The model under review builds one solid part; all positions refer to its coordinate system, in mm. A direction names the side the tool comes from. Round coordinates to 2 decimals unless told otherwise and drop trailing zeros. Loops run counter-clockwise (first coordinate to the right, second up) from the corner with the lowest first, then second, coordinate; pieces in that order, holes last. Notation, with made-up numbers: M 42,-17.5 L 47,-17.5 A27 ccw 47,-1.5 Z; hole C 25.5,51.25 d2. An arc over 180 degrees is marked long. Return JSON: item names as keys, results as strings. Group by question number.
Q1. For faces 1 (the face through (-14, 22.5, 0)), 2 (the face through (-11.5, 10, 0)), 3 (the face through (-3.32, 28.7, 0.95)), list the 3-axis set-ups (+Z, -Z, +X, -X, +Y, -Y) from which the entire face can be reached by the end or side of a thin tool; tool diameter is ignored.
Q2. To check wall thickness, follow line 1 along Y through (x, z) = (-0.5, -1.25); line 2 along X through (y, z) = (15, 4); line 3 along Y through (x, z) = (-13.5, -5.5). State the ranges of each line that lie inside material, in increasing order.
Q3. Clearance check with flat-ended pins moving along their axes: pin 1 Ø2 at (x, z) = (-14.5, -3) entering from -Y; pin 2 Ø3.5 at (y, z) = (24.5, -2) entering from -X; pin 3 Ø3.5 at (x, z) = (-12.5, 1) entering from +Y. State where each tip first meets the part, or that it passes through.
Q4. Consider section D-D (y = 18.5). State the section outline as (x, z) points, and give its area (3 significant figures).
Q5. Consider section C-C (z = 0). State the section outline as (x, y) points (3 decimals), and give its area (3 significant figures).
Q6. Consider section B-B (x = -6.35). State the section outline as (y, z) points (3 decimals).
Q7. Consider section A-A (z = 5). State the section outline as (x, y) points.
Autodesk Inventor part; units mm, degrees
ref_plane "YZ Plane" through (0, 0, 0) normal (1, 0, 0) x (0, 1, 0)
ref_plane "XZ Plane" through (0, 0, 0) normal (0, 1, 0) x (-1, 0, 0)
ref_plane "XY Plane" through (0, 0, 0) normal (0, 0, 1) x (1, 0, 0)
sketch "Sketch1" plane through (0, 0, 0) normal (0, 1, 0) x (-1, 0, 0)
  line L0 (11.5, -6) -> (-11.5, -6)
  line L1 (-11.5, -6) -> (-11.5, 6)
  line L2 (-11.5, 6) -> (11.5, 6)
  line L3 (11.5, 6) -> (11.5, -6)
  line L4 (11.5, -6) -> (-11.5, 6) construction
  line L5 (-11.5, -6) -> (11.5, 6) construction
  point P0 (0, 0)
  dimension "d0" = 23
  dimension "d1" = 12
extrude "Extrusion1" add sketch "Sketch1" along normal blind 19.5
sketch "Sketch2" plane through (0, 19.5, 0) normal (0, 1, 0) x (1, 0, 0)
  line L0 (16, -6) -> (-16, -6)
  line L1 (-16, -6) -> (-16, 6)
  line L2 (-16, 6) -> (16, 6)
  line L3 (16, 6) -> (16, -6)
  line L4 (16, -6) -> (-16, 6) construction
  line L5 (-16, -6) -> (16, 6) construction
  point P0 (0, 0)
  dimension "d4" = 32
  dimension "d5" = 12
extrude "Extrusion2" add sketch "Sketch2" along normal blind 3
sketch "Sketch3" plane through (0, 22.5, 0) normal (0, 1, 0) x (1, 0, 0)
  line L0 (11.5, 6) -> (16, 6)
  line L1 (-11.5, -6) -> (11.5, -6)
  line L2 (11.5, -6) -> (11.5, 6)
  line L3 (11.5, 6) -> (-11.5, 6)
  line L4 (-11.5, 6) -> (-11.5, -6)
  line L5 (-11.5, -6) -> (11.5, 6) construction
  line L6 (11.5, -6) -> (-11.5, 6) construction
  point P0 (0, 0)
extrude "Extrusion3" add sketch "Sketch3" along normal blind 3
sketch "Sketch4" plane through (0, 25.5, 0) normal (0, 1, 0) x (1, 0, 0)
  circle A0 centre (-6.35, 0) radius 3.175
  point P0 (0, 0)
  dimension "d10" = 6.35
extrude "Extrusion4" add sketch "Sketch4" along normal blind 6.5
properties part number "sg90_servo"
Values:
{
 "1": {"face 1": "+Z, -Z, -X, +Y", "face 2": "+Z, -Z, -X, -Y", "face 3": "+Y"},
 "2": {"line 1": "y = 0 to 25.5", "line 2": "x = -11.5 to 11.5", "line 3": "y = 19.5 to 22.5"},
 "3": {"pin 1": "stops at y = 19.5", "pin 2": "stops at x = -11.5", "pin 3": "stops at y = 25.5"},
 "4": {"outline": "M -11.5,-6 L 11.5,-6 L 11.5,6 L -11.5,6 Z", "area": "276 mm2"},
 "5": {"outline": "M -16,19.5 L -11.5,19.5 L -11.5,0 L 11.5,0 L 11.5,19.5 L 16,19.5 L 16,22.5 L 11.5,22.5 L 11.5,25.5 L -3.175,25.5 L -3.175,32 L -9.525,32 L -9.525,25.5 L -11.5,25.5 L -11.5,22.5 L -16,22.5 Z", "area": "655 mm2"},
 "6": {"outline": "M 0,-6 L 25.5,-6 L 25.5,-3.175 L 32,-3.175 L 32,3.175 L 25.5,3.175 L 25.5,6 L 0,6 Z"},
 "7": {"outline": "M -16,19.5 L -11.5,19.5 L -11.5,0 L 11.5,0 L 11.5,19.5 L 16,19.5 L 16,22.5 L 11.5,22.5 L 11.5,25.5 L -11.5,25.5 L -11.5,22.5 L -16,22.5 Z"}
}
